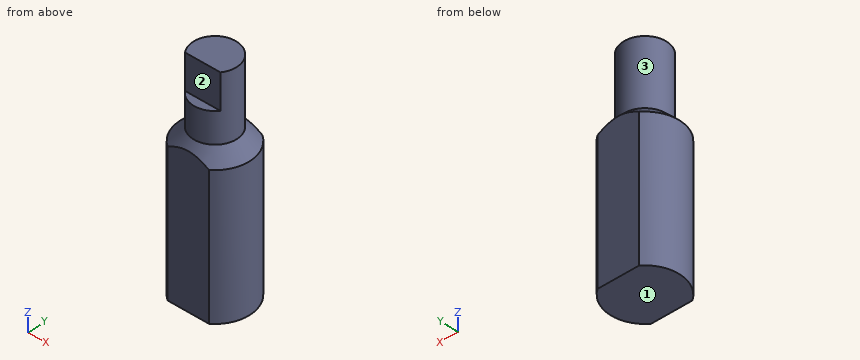
```python
from build123d import *

# Parameters (mm, degrees)
F3_W     = 20
F3_H     = 8
F4_DEPTH = 10
F5_W     = 19.943191
F5_H     = 60
F6_DEPTH = 12.5


with BuildPart() as f1:
    # F0 (on Front) → F1 (revolve)
    with BuildSketch(Plane.XZ):
        Polygon((5, 0), (0, 0), (0, -50), (8, -50), (8, -18), (5, -15), align=None)
    revolve(axis=Axis((0, 0, -25), (0, 0, 1)))

    # F3 (on offset) → F4 (cut)
    with BuildSketch(Plane.XZ.offset(3)):
        with Locations((-0.236336, -4)):
            Rectangle(F3_W, F3_H)
    extrude(amount=F4_DEPTH, mode=Mode.SUBTRACT)

    # F5 (on Right) → F6 (cut, symmetric)
    with BuildSketch(Plane.YZ):
        with Locations((16.471595, -30)):
            Rectangle(F5_W, F5_H)
        with Locations((-16.471595, -30)):
            Rectangle(F5_W, F5_H)
    extrude(amount=F6_DEPTH, both=True, mode=Mode.SUBTRACT)


solid = f1.part
```
Source: CAD feature listing. Evaluate the final solid. Frame: model axes, mm. Face numbers are marked on the shaded views. A direction names the side the tool comes from. Round coordinates to 2 decimals unless told otherwise and drop trailing zeros. Loops run counter-clockwise (first coordinate to the right, second up) from the corner with the lowest first, then second, coordinate; pieces in that order, holes last. Notation, with made-up numbers: M 70,-12.75 L 77,-12.75 A21 ccw 77,5.25 Z; hole C 55,-35 d6. An arc over 180 degrees is marked long. Use a Markdown table: item, result. Add a question column.
1. Cut plane B-B, the plane y = 0. Output: boundary loops of the cut face in (x, z), and give its area (3 significant figures).
2. Ray query, line 1 along Y through (x, z) = (6.5, -45.5); line 2 along Z through (x, y) = (-5, 3.5); line 3 along Z through (x, y) = (7.25, -0.25). Return the intervals inside material, ascending. Write a range as [from, to].
3. Cut plane C-C, the plane z = -11. Output: boundary loops of the cut face in (x, y), and give its area (3 significant figures).
4. Contact query for flat-ended pins moving along their axis: pin 1 (4 mm diameter, centred on y = 3, z = -15, fed in from +X); pin 2 (6 mm diameter, centred on y = 5, z = -25, fed in from +X); pin 3 (1 mm diameter, centred on y = 3.5, z = -27, fed in from +X); pin 4 (1 mm diameter, centred on y = -0.5, z = -41.5, fed in from +X). Output: stop coordinate, or through.
5. Cut plane D-D, the plane z = -41. Output: boundary loops of the cut face in (x, y), and give its area (3 significant figures).
6. Cut plane A-A, the plane x = 0. Output: boundary loops of the cut face in (y, z).
7. Set-up query: the marked faces 1, 2 and 3. Return all of +Z, -Z, +X, -X, +Y, -Y with unobstructed straight access to the full face (end or side cutting, diameter ignored); none if empty.
Solution:
| question | item | result |
|---|---|---|
| 1 | outline | M -8,-50 L 8,-50 L 8,-18 L 5,-15 L 5,0 L -5,0 L -5,-15 L -8,-18 Z |
| 1 | area | 701 mm2 |
| 2 | line 1 | y = [-4.66, 4.66] |
| 2 | line 2 | z = [-50, -16.1] |
| 2 | line 3 | z = [-50, -17.25] |
| 3 | outline | C 0,0 d10 |
| 3 | area | 78.5 mm2 |
| 4 | pin 1 | stops at x = 6.48 |
| 4 | pin 2 | stops at x = 7.75 |
| 4 | pin 3 | stops at x = 7.42 |
| 4 | pin 4 | stops at x = 8 |
| 5 | outline | M -4.66,-6.5 L 4.66,-6.5 A8 ccw 4.66,6.5 L -4.66,6.5 A8 ccw Z |
| 5 | area | 182 mm2 |
| 6 | outline | M -6.5,-50 L 6.5,-50 L 6.5,-16.5 L 5,-15 L 5,0 L -3,0 L -3,-8 L -5,-8 L -5,-15 L -6.5,-16.5 Z |
| 7 | face 1 | -Z, +X, -X, +Y, -Y |
| 7 | face 2 | +Z, +X, -X, -Y |
| 7 | face 3 | +Z |
